```python
from build123d import *

# Parameters (mm, degrees)
SKETCH1_R               = 1.5
BOSS_EXTRUDE1_DEPTH     = 3
CUT_EXTRUDE1_DEPTH      = 56.407580709
CUT_EXTRUDE1_DEPTH_BACK = 56.407580709
CUT_EXTRUDE2_DEPTH      = 54.918920612
CUT_EXTRUDE2_DEPTH_BACK = 54.918920612
CHAMFER1_SIZE           = 1


with BuildPart() as part:
    # Sketch1 → Boss-Extrude1 (new body)
    with BuildSketch(Plane(origin=(0, 0, 0), x_dir=(1, 0, 0), z_dir=(0, 1, 0))):
        Polygon((-55, 3), (-52, 6), (52, 6), (55, 3), (55, -3), (52, -6), (-52, -6), (-55, -3), align=None)
        with Locations(Location((-50, 0, 0), (0, 0, 270))):
            Circle(SKETCH1_R, mode=Mode.SUBTRACT)
        with Locations(Location((0, 0, 0), (0, 0, 270))):
            Circle(SKETCH1_R, mode=Mode.SUBTRACT)
        with Locations(Location((50, 0, 0), (0, 0, 270))):
            Circle(SKETCH1_R, mode=Mode.SUBTRACT)
    extrude(amount=BOSS_EXTRUDE1_DEPTH)

    # Sketch2 → Cut-Extrude1 (cut, two sides: drawn at the far end of the back side and taken through both)
    with BuildSketch(Plane(origin=(0, 3, 0), x_dir=(1, 0, 0), z_dir=(0, 1, 0)).offset(-CUT_EXTRUDE1_DEPTH_BACK)):
        Polygon((-53.5, 4.5), (-53.5, -4.5), (-55, -3), (-55, 3), align=None)
        Polygon((53.5, -4.5), (55, -3), (55, 3), (53.5, 4.5), align=None)
    extrude(amount=CUT_EXTRUDE1_DEPTH + CUT_EXTRUDE1_DEPTH_BACK, mode=Mode.SUBTRACT)

    # Sketch3 → Cut-Extrude2 (cut, two sides: drawn at the far end of the back side and taken through both)
    with BuildSketch(Plane(origin=(0, 3, 0), x_dir=(1, 0, 0), z_dir=(0, 1, 0)).offset(-CUT_EXTRUDE2_DEPTH_BACK)):
        Polygon((-49, -6), (-53.5, -1.5), (-53.5, -4.5), (-52, -6), align=None)
        Polygon((-53.5, 4.5), (-53.5, 1.5), (-49, 6), (-52, 6), align=None)
        Polygon((52, 6), (49, 6), (53.5, 1.5), (53.5, 4.5), align=None)
        Polygon((53.5, -1.5), (49, -6), (52, -6), (53.5, -4.5), align=None)
    extrude(amount=CUT_EXTRUDE2_DEPTH + CUT_EXTRUDE2_DEPTH_BACK, mode=Mode.SUBTRACT)

    # Chamfer1
    chamfer1_edges = [part.edges().sort_by_distance(p)[0] for p in [
        (49, 1.5, -6),
        (53.5, 1.5, -1.5),
        (-53.5, 1.5, -1.5),
        (-49, 1.5, -6),
        (-49, 1.5, 6),
        (-53.5, 1.5, 1.5),
        (53.5, 1.5, 1.5),
        (49, 1.5, 6),
    ]]
    chamfer(chamfer1_edges, length=CHAMFER1_SIZE)


solid = part.part
```
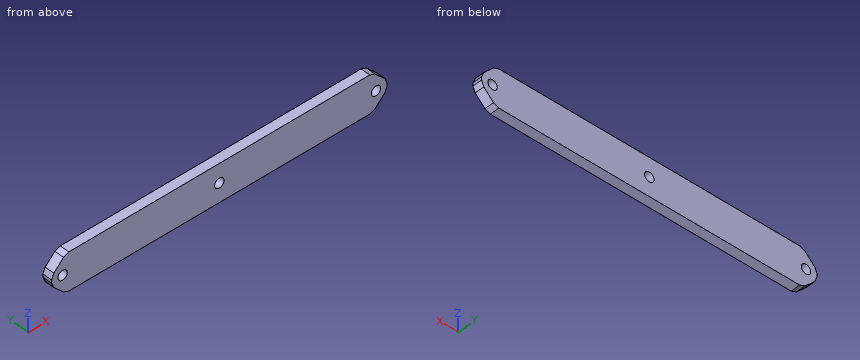
The listing builds one solid part. Answer for the finished solid, in the listing's coordinates (mm). Give positions to 0.01 mm unless a question says otherwise; leave off trailing zeros. Write each loop counter-clockwise with the first axis right and the second up, starting at its lowest first coordinate (ties: lowest second). Pieces come first, ordered by that corner, then holes. Notation, with made-up numbers: (80.5, 74.5) -> (92.5, 74.5) arc R29 cw to (92.5, 108.5) -> close; hole circle Ø4 at (14, -9.5). An arc over 180 degrees is marked (long way). Write item = value, one per line. Start each with the question number.
1) The part is cut by section B-B, the plane y = 2.2. Determine the outline of the cut face in (x, z), and give its area (3 significant figures).
2) The part is cut by section A-A, the plane x = 0. Determine the outline of the cut face in (y, z), and give its area (3 significant figures).
3) Straight lines are drawn through the part: line 1 along X through (y, z) = (0.9, 0); line 2 along X through (y, z) = (0.8, 1.25); line 3 along X through (y, z) = (0.95, -2.25). For each, find the intervals that lie inside material, in ascending order.
4) This flat-tipped pin is pushed along its axis until it touches: pin 1 (2.5 mm diameter, centred on x = 50, z = 0, fed in from -Y). Where does it stop, or does it pass through?
Solutions:
q1.outline = (-53.5, -0.5) -> (-52.79, -2.21) -> (-49.71, -5.29) -> (-48, -6) -> (48, -6) -> (49.71, -5.29) -> (52.79, -2.21) -> (53.5, -0.5) -> (53.5, 0.5) -> (52.79, 2.21) -> (49.71, 5.29) -> (48, 6) -> (-48, 6) -> (-49.71, 5.29) -> (-52.79, 2.21) -> (-53.5, 0.5) -> close; hole circle Ø3 at (-50, 0); hole circle Ø3 at (0, 0); hole circle Ø3 at (50, 0)
q1.area = 1,220 mm²
q2.outline = (0, -6) -> (3, -6) -> (3, -1.5) -> (0, -1.5) -> close; (0, 1.5) -> (3, 1.5) -> (3, 6) -> (0, 6) -> close
q2.area = 27.0 mm²
q3.line_1 = -53.5 to -51.5, -48.5 to -1.5, 1.5 to 48.5, 51.5 to 53.5
q3.line_2 = -53.19 to -50.83, -49.17 to -0.83, 0.83 to 49.17, 50.83 to 53.19
q3.line_3 = -52.75 to 52.75
q4.pin_1 = through
